from build123d import *

# Parameters (mm, degrees)
F0_W      = 52.3875
F0_H      = 31.75
F1_DEPTH  = 3.175
F3_DEPTH  = 3.176
F4_R      = 3.5687
F5_DEPTH  = 9.525
F6_R      = 2.778125
F7_DEPTH  = 12.701
F9_DEPTH  = 9.525
F10_R     = 3.175
F11_DEPTH = 3.176


with BuildPart() as f1:
    # F0 (on Front) → F1 (new body)
    with BuildSketch(Plane.XZ):
        with Locations((1.981661, -8.707554)):
            Rectangle(F0_W, F0_H)
    extrude(amount=F1_DEPTH)

    # F2 (on face) → F3 (cut, through all)
    with BuildSketch(Plane.XZ.offset(3.175)):
        with BuildLine():
            ThreePointArc((-14.290214, 0.817446), (-17.862089, 4.389321), (-21.433964, 0.817446))
            ThreePointArc((-21.433964, 0.817446), (-17.862089, -2.754429), (-14.290214, 0.817446))
        make_face()
    extrude(amount=-F3_DEPTH, mode=Mode.SUBTRACT)

    # F4 (on face) → F5 (join)
    with BuildSketch(Plane.XZ.offset(3.175)):
        with Locations((21.825411, 0.817446)):
            Circle(F4_R)
    extrude(amount=F5_DEPTH)

    # F6 (on face) → F7 (cut, through all)
    with BuildSketch(Plane.XZ.offset(12.7)):
        with Locations((21.825411, 0.817446)):
            Circle(F6_R)
    extrude(amount=-F7_DEPTH, mode=Mode.SUBTRACT)

    # F8 (on face) → F9 (join)
    with BuildSketch(Plane.XZ.offset(3.175)):
        with BuildLine():
            ThreePointArc((-14.687089, -18.232554), (-17.862089, -15.057554), (-21.037089, -18.232554))
            ThreePointArc((-21.037089, -18.232554), (-17.862089, -21.407554), (-14.687089, -18.232554))
        make_face()
    extrude(amount=F9_DEPTH)

    # F10 (on face) → F11 (cut, through all)
    with BuildSketch(Plane.XZ.offset(3.175)):
        with Locations((21.825411, -18.232554)):
            Circle(F10_R)
    extrude(amount=-F11_DEPTH, mode=Mode.SUBTRACT)


solid = f1.part
For this review, take the finished solid that the model builds, in its own axes (mm). A direction names the side the tool comes from. Round coordinates to 2 decimals unless told otherwise and drop trailing zeros. Write each loop counter-clockwise with the first axis right and the second up, starting at its lowest first coordinate (ties: lowest second). Pieces come first, ordered by that corner, then holes. Notation, with made-up numbers: (-12.5, -12) - (15.5, -12) arc R19 cw to (15.5, 7) - close; hole circle Ø2 at (67.25, -1). An arc over 180 degrees is marked (long way). Write item = value, one per line. Start each with the question number.
1. Consider section C-C on z = -17. State the section outline as (x, y) points (3 decimals).
2. Consider section D-D on z = 3. State the section outline as (x, y) points (3 decimals).
3. Consider section B-B on y = -6.5. State the section outline as (x, z) points (3 decimals).
4. Consider section A-A on x = 21. State the section outline as (y, z) points (3 decimals), plus the area to 3 significant figures.
5. Draft analysis for pull direction Z (two halves, no side actions). For faces 3 (the face through (2, -2, 7.167)), 4 (the face through (2, 0, -8)), 5 (the face through (19.05, -6.44, 0.94)), 6 (the face through (21.137, -1.61, -21.332)), state which applies: released by +Z, released by -Z, zero draft, split by the parting line, or undercut.
6. For faces 1 (the face through (-17.174, -7.871, -15.133)), 2 (the face through (2, -2, -24.583)), list the 3-axis set-ups (+Z, -Z, +X, -X, +Y, -Y) from which the entire face can be reached by the end or side of a thin tool; tool diameter is ignored.
7. For pin 1 Ø5.5 at (x, z) = (21.83, -18.23) entering from +Y; pin 2 Ø12 at (x, z) = (10, -18.5) entering from -Y (3 decimals); pin 3 Ø3 at (y, z) = (-8.5, -1) entering from +X; pin 4 Ø3 at (y, z) = (-10, 3) entering from -X, all flat-tipped, find the tip position at first contact; note any pin that passes through.
8. Wall thickness on L1, parallel to X at y = -1.75, z = 1; L2, parallel to Z at x = -18, y = -1.75; L3, parallel to X at y = -8, z = 1: over which ranges is each line inside the solid? List them lowest first.
Evaluation:
q1.outline = (-24.212, -3.175) - (-20.788, -3.175) - (-20.788, -12.7) - (-14.936, -12.7) - (-14.936, -3.175) - (18.899, -3.175) - (18.899, 0) - (-24.212, 0) - close; (24.751, -3.175) - (28.175, -3.175) - (28.175, 0) - (24.751, 0) - close
q2.outline = (-24.212, -3.175) - (-20.69, -3.175) - (-20.69, 0) - (-24.212, 0) - close; (-15.035, -3.175) - (19.002, -3.175) - (19.002, -12.7) - (20.107, -12.7) - (20.107, 0) - (-15.035, 0) - close; (23.544, -12.7) - (24.649, -12.7) - (24.649, -3.175) - (28.175, -3.175) - (28.175, 0) - (23.544, 0) - close
q3.outline = circle Ø6.35 at (-17.862, -18.233); circle Ø7.137 at (21.825, 0.817); hole circle Ø5.556 at (21.825, 0.817)
q4.outline = (-12.7, -2.654) - (-3.175, -2.654) - (-3.175, -15.167) - (0, -15.167) - (0, -1.835) - (-12.7, -1.835) - close; (-12.7, 3.47) - (0, 3.47) - (0, 7.167) - (-3.175, 7.167) - (-3.175, 4.289) - (-12.7, 4.289) - close; (-3.175, -24.583) - (0, -24.583) - (0, -21.298) - (-3.175, -21.298) - close
q4.area = 80.1 mm2
q5.face_3 = released by +Z
q5.face_4 = zero draft
q5.face_5 = undercut
q5.face_6 = undercut
q6.face_1 = -Y
q6.face_2 = -Z, +X, -X, +Y, -Y
q7.pin_1 = through
q7.pin_2 = -3.175
q7.pin_3 = 25.38
q7.pin_4 = 18.32
q8.L1 = -24.21 to -21.43, -14.29 to 19.05, 24.6 to 28.18
q8.L2 = -24.58 to -2.75, 4.39 to 7.17
q8.L3 = 18.26 to 19.05, 24.6 to 25.39
